```python
from build123d import *

# Parameters (mm, degrees)
SKETCH1_R           = 11.4046
SKETCH1_R_2         = 8.382
BOSS_EXTRUDE1_DEPTH = 6.35
SKETCH1_3_R         = 8.382
SKETCH1_3_R_2       = 3.175
BOSS_EXTRUDE2_DEPTH = 13.97
SKETCH1_4_R         = 9.398
SKETCH1_4_R_2       = 8.382
CUT_EXTRUDE1_DEPTH  = 1.778
CUT_EXTRUDE3_START  = 6.35
SKETCH1_8_R         = 9.398
SKETCH1_8_R_2       = 8.382
CUT_EXTRUDE3_DEPTH  = 1.778
BOSS_EXTRUDE3_DEPTH = 6.35
CIRPATTERN1_COUNT   = 24


with BuildPart() as part:
    # Sketch1 → Boss-Extrude1 (new body)
    with BuildSketch(Plane(origin=(0, 0, 0), x_dir=(1, 0, 0), z_dir=(0, 1, 0))):
        Circle(SKETCH1_R)
        Circle(SKETCH1_R_2, mode=Mode.SUBTRACT)
    extrude(amount=BOSS_EXTRUDE1_DEPTH)

    # Sketch1_3 → Boss-Extrude2 (add)
    with BuildSketch(Plane(origin=(0, 0, 0), x_dir=(1, 0, 0), z_dir=(0, 1, 0))):
        Circle(SKETCH1_3_R)
        Circle(SKETCH1_3_R_2, mode=Mode.SUBTRACT)
    extrude(amount=BOSS_EXTRUDE2_DEPTH)

    # Sketch1_4 → Cut-Extrude1 (cut)
    with BuildSketch(Plane(origin=(0, 0, 0), x_dir=(1, 0, 0), z_dir=(0, 1, 0))):
        Circle(SKETCH1_4_R)
        Circle(SKETCH1_4_R_2, mode=Mode.SUBTRACT)
    extrude(amount=CUT_EXTRUDE1_DEPTH, mode=Mode.SUBTRACT)

    # Sketch1_8 → Cut-Extrude3 (cut)
    with BuildSketch(Plane(origin=(0, 0, 0), x_dir=(1, 0, 0), z_dir=(0, 1, 0)).offset(CUT_EXTRUDE3_START)):
        Circle(SKETCH1_8_R)
        Circle(SKETCH1_8_R_2, mode=Mode.SUBTRACT)
    extrude(amount=-CUT_EXTRUDE3_DEPTH, mode=Mode.SUBTRACT)

    # Sketch2 → Boss-Extrude3 (add)
    with BuildSketch(Plane(origin=(0, 6.35, 0), x_dir=(1, 0, 0), z_dir=(0, 1, 0))):
        with BuildLine():
            Line((0.3772543, 13.715999489), (-0.3847457, 13.715999489))
            Line((-0.3847457, 13.715999489), (-1.145852444, 11.34689047))
            ThreePointArc((-1.145852444, 11.34689047), (-0.002866915, 11.40459964), (1.140147484, 11.34746513))
            Line((1.140147484, 11.34746513), (0.3772543, 13.715999489))
        make_face()
    boss_extrude3 = extrude(amount=-BOSS_EXTRUDE3_DEPTH)

    # CirPattern1: Boss-Extrude3 ×24 about axis
    cirpattern1_axis = Axis((0, 0, 0), (0, 1, 0))
    for i in range(1, CIRPATTERN1_COUNT):
        add(boss_extrude3.rotate(cirpattern1_axis, i * 360 / CIRPATTERN1_COUNT))


solid = part.part
```
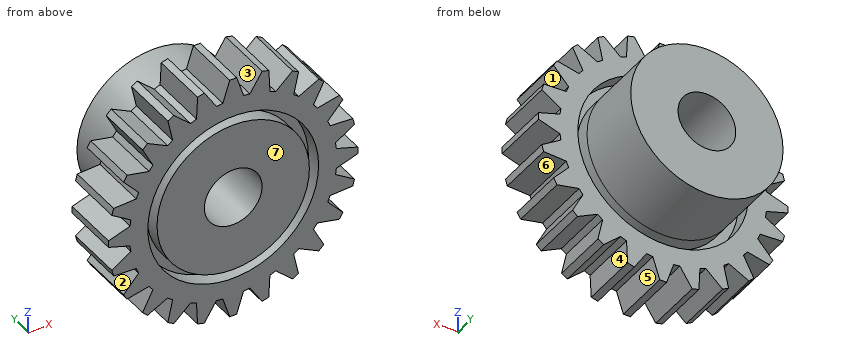
For this review, take the finished solid that the model builds, in its own axes (mm). Face numbers are marked on the shaded views. A direction names the side the tool comes from. Round coordinates to 2 decimals unless told otherwise and drop trailing zeros. Write each loop counter-clockwise with the first axis right and the second up, starting at its lowest first coordinate (ties: lowest second). Pieces come first, ordered by that corner, then holes. Notation, with made-up numbers: (29, 84) -> (48, 84) arc R28 ccw to (48, 103) -> close; hole circle Ø10 at (-20.5, 79.5). An arc over 180 degrees is marked (long way). One line per question, with ' | ' between items. Start each with the question number.
(1) Add section D-D, the plane y = 10. Write out the cut boundary in (x, z) (3 decimals).
(2) Add section B-B, the plane z = 0. Write out the cut boundary in (x, y) (3 decimals), plus the area to 3 significant figures.
(3) For line 1 along X through (y, z) = (0.6, 0) (3 decimals); line 2 along X through (y, z) = (4.25, -11.75), list the stretches that pass through material, from the lowest coordinate up. Write a range as from..to.
(4) Insertion check: P1, Ø3, axis at x = 6.5, y = 7.5, coming from the -Z side; P2, Ø2, axis at x = 7, z = -10.5, coming from the +Y side. Each pin has a flat end and moves straight along its axis. Give the tip position at first contact, or say it passes through.
(5) Tool access review of the marked faces 1, 2 and 3: name each direction out of +Z, -Z, +X, -X, +Y, -Y from which nothing blocks a thin tool from reaching the whole face with its end or side.
(6) Add section C-C, the plane y = 5. Give the number of separate pieces and of enclosed holes in the cut face, plus the area to 3 significant figures.
(7) Add section A-A, the plane x = 0. Write out the cut boundary in (y, z) (3 decimals).
(8) Mouldability with a two-part tool opening along X and no side actions: class the marked faces 4, 5, 6 and 7 as released by +X, released by -X, zero draft, split by the parting line, or undercut.
Answer list:
1) outline: circle Ø16.764 at (0, 0); hole circle Ø6.35 at (0, 0)
2) outline: (-13.716, 0) -> (-9.398, 0) -> (-9.398, 1.778) -> (-8.382, 1.778) -> (-8.382, 0) -> (-3.175, 0) -> (-3.175, 13.97) -> (-8.382, 13.97) -> (-8.382, 4.572) -> (-9.398, 4.572) -> (-9.398, 6.35) -> (-13.716, 6.35) -> close; (3.175, 0) -> (8.382, 0) -> (8.382, 1.778) -> (9.398, 1.778) -> (9.398, 0) -> (13.716, 0) -> (13.716, 6.35) -> (9.398, 6.35) -> (9.398, 4.572) -> (8.382, 4.572) -> (8.382, 13.97) -> (3.175, 13.97) -> close | area: 206 mm²
3) line 1: -13.716..-9.398, -8.382..-3.175, 3.175..8.382, 9.398..13.716 | line 2: -7.08..-6.18, -3.99..-2.15, -1.02..1.01, 2.15..3.98, 6.17..7.08
4) P1: z = -12.07 | P2: y = 6.35
5) face 1: +X, +Y, -Y | face 2: -X, +Y, -Y | face 3: +Z, +Y, -Y
6) separate pieces: 2 | enclosed holes: 2 | area: 405 mm²
7) outline: (0, -13.716) -> (6.35, -13.716) -> (6.35, -9.398) -> (4.572, -9.398) -> (4.572, -8.382) -> (13.97, -8.382) -> (13.97, -3.175) -> (0, -3.175) -> (0, -8.382) -> (1.778, -8.382) -> (1.778, -9.398) -> (0, -9.398) -> close; (0, 3.175) -> (13.97, 3.175) -> (13.97, 8.382) -> (4.572, 8.382) -> (4.572, 9.398) -> (6.35, 9.398) -> (6.35, 13.716) -> (0, 13.716) -> (0, 9.398) -> (1.778, 9.398) -> (1.778, 8.382) -> (0, 8.382) -> close
8) face 4: undercut | face 5: undercut | face 6: released by +X | face 7: zero draft
